For this review, take the finished solid that the model builds, in its own axes (mm). Face numbers are marked on the shaded views. Coordinates: 2 decimals unless noted, no trailing zeros.
from build123d import *

# Parameters (mm, degrees)
SKETCH1_W              = 457.2
SKETCH1_H              = 406.4
BOSS_EXTRUDE1_DEPTH    = 12.7
F_6_CLEARANCE_HOLE1_D  = 3.7973
SKETCH5_R              = 6.4135
CUT_EXTRUDE2_DEPTH     = 307.120058147
CUT_EXTRUDE3_DEPTH     = 3.175
F_10_CLEARANCE_HOLE1_D = 5.1054
CUT_EXTRUDE4_DEPTH     = 307.120058147
FILLET1_R              = 6.35
F_10_CLEARANCE_HOLE2_D = 5.1054
SKETCH18_R             = 6.985
CUT_EXTRUDE6_DEPTH     = 4.7625


with BuildPart() as part:
    # Sketch1 → Boss-Extrude1 (new body)
    with BuildSketch(Plane(origin=(0, 0, 0), x_dir=(1, 0, 0), z_dir=(0, 1, 0))):
        Rectangle(SKETCH1_W, SKETCH1_H)
    extrude(amount=BOSS_EXTRUDE1_DEPTH)

    # #6 Clearance Hole1 (through all)
    with Locations(Plane(origin=(0, 0, 0), x_dir=(-1, 0, 0), z_dir=(0, -1, 0))):
        with Locations((-196.85, 87.87638), (-158.75, 87.87638), (-146.05, 90.45448), (-107.95, 90.45448), (-95.25, 95.83166), (-57.15, 95.83166), (-44.45, 101.50348), (-6.35, 101.50348), (6.35, 107.61726), (44.45, 107.61726), (57.15, 110.71098), (95.25, 110.71098), (107.95, 117.34038), (146.05, 117.34038), (158.75, 124.26442), (196.85, 124.26442), (196.85, -124.26442), (158.75, -124.26442), (146.05, -117.34038), (107.95, -117.34038), (95.25, -110.71098), (57.15, -110.71098), (44.45, -107.61726), (6.35, -107.61726), (-6.35, -101.50348), (-44.45, -101.50348), (-57.15, -95.83166), (-95.25, -95.83166), (-107.95, -90.45448), (-146.05, -90.45448), (-158.75, -87.87638), (-196.85, -87.87638)):
            Hole(F_6_CLEARANCE_HOLE1_D / 2)

    # Sketch5 → Cut-Extrude2 (cut, through all)
    with BuildSketch(Plane.XZ):
        with Locations(Location((0, 0, 0), (0, 0, 270))):
            Circle(SKETCH5_R)
    extrude(amount=-CUT_EXTRUDE2_DEPTH, mode=Mode.SUBTRACT)

    # Sketch6 → Cut-Extrude3 (cut)
    with BuildSketch(Plane.XZ):
        Polygon((-192.913, -121.99139199), (-196.85, -119.71836398), (-200.787, -121.99139199), (-200.787, -126.53744801), (-196.85, -128.81047602), (-192.913, -126.53744801), align=None)
    cut_extrude3 = extrude(amount=-CUT_EXTRUDE3_DEPTH, mode=Mode.SUBTRACT)

    # Sketch-Pattern1: Cut-Extrude3 at 31 more places
    with Locations((393.7, 0, 36.38804), (355.6, 0, 36.38804), (342.9, 0, 33.80994), (304.8, 0, 33.80994), (292.1, 0, 28.43276), (254, 0, 28.43276), (241.3, 0, 22.76094), (203.2, 0, 22.76094), (190.5, 0, 16.64716), (152.4, 0, 16.64716), (139.7, 0, 13.55344), (101.6, 0, 13.55344), (88.9, 0, 6.92404), (50.8, 0, 6.92404), (38.1, 0, 0), (0, 0, 248.52884), (38.1, 0, 248.52884), (50.8, 0, 241.6048), (88.9, 0, 241.6048), (101.6, 0, 234.9754), (139.7, 0, 234.9754), (152.4, 0, 231.88168), (190.5, 0, 231.88168), (203.2, 0, 225.7679), (241.3, 0, 225.7679), (254, 0, 220.09608), (292.1, 0, 220.09608), (304.8, 0, 214.7189), (342.9, 0, 214.7189), (355.6, 0, 212.1408), (393.7, 0, 212.1408)):
        add(cut_extrude3, mode=Mode.SUBTRACT)

    # #10 Clearance Hole1 (through all)
    with Locations(Plane(origin=(0, 12.7, 0), x_dir=(1, 0, 0), z_dir=(0, 1, 0))):
        with Locations((-30.245937227, -17.4625), (0, 34.925), (30.245937227, -17.4625)):
            Hole(F_10_CLEARANCE_HOLE1_D / 2)

    # Sketch10 → Cut-Extrude4 (cut, through all)
    with BuildSketch(Plane(origin=(0, 12.7, 0), x_dir=(1, 0, 0), z_dir=(0, 1, 0))):
        Polygon((67.035234154, -203.2), (228.6, -171.45), (228.6, -203.2), align=None)
        Polygon((228.6, 203.2), (67.035234154, 203.2), (228.6, 171.45), align=None)
    extrude(amount=-CUT_EXTRUDE4_DEPTH, mode=Mode.SUBTRACT)

    # Fillet1
    fillet1_edges = [part.edges().sort_by_distance(p)[0] for p in [
        (67.035234154, 6.35, 203.2),
        (228.6, 6.35, 171.45),
        (228.6, 6.35, -171.45),
        (67.035234154, 6.35, -203.2),
        (-228.6, 6.35, 203.2),
        (-228.6, 6.35, -203.2),
    ]]
    fillet(fillet1_edges, radius=FILLET1_R)

    # #10 Clearance Hole2 (through all)
    with Locations(Plane(origin=(0, 12.7, 0), x_dir=(1, 0, 0), z_dir=(0, 1, 0))):
        with Locations((177.8, -129.661378082), (-177.8, -152.4), (-177.8, 152.4), (177.8, 129.661378082)):
            Hole(F_10_CLEARANCE_HOLE2_D / 2)

    # Sketch18 → Cut-Extrude6 (cut)
    with BuildSketch(Plane.XZ):
        with Locations(Location((-196.85, -124.26442, 0), (0, 0, 270))):
            Circle(SKETCH18_R)
    cut_extrude6 = extrude(amount=-CUT_EXTRUDE6_DEPTH, mode=Mode.SUBTRACT)

    # Sketch-Pattern2: Cut-Extrude6 at 31 more places
    with Locations((393.7, 0, 36.38804), (355.6, 0, 36.38804), (342.9, 0, 33.80994), (304.8, 0, 33.80994), (292.1, 0, 28.43276), (254, 0, 28.43276), (241.3, 0, 22.76094), (203.2, 0, 22.76094), (190.5, 0, 16.64716), (152.4, 0, 16.64716), (139.7, 0, 13.55344), (101.6, 0, 13.55344), (88.9, 0, 6.92404), (50.8, 0, 6.92404), (38.1, 0, 0), (0, 0, 248.52884), (38.1, 0, 248.52884), (50.8, 0, 241.6048), (88.9, 0, 241.6048), (101.6, 0, 234.9754), (139.7, 0, 234.9754), (152.4, 0, 231.88168), (190.5, 0, 231.88168), (203.2, 0, 225.7679), (241.3, 0, 225.7679), (254, 0, 220.09608), (292.1, 0, 220.09608), (304.8, 0, 214.7189), (342.9, 0, 214.7189), (355.6, 0, 212.1408), (393.7, 0, 212.1408)):
        add(cut_extrude6, mode=Mode.SUBTRACT)


solid = part.part
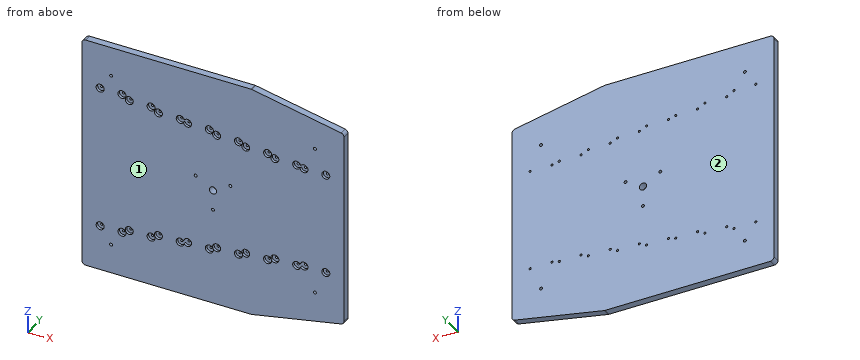
1. Clearance check with flat-ended pins moving along their axes: pin 1 Ø3 at (x, z) = (-13.5, -89.5) entering from -Y; pin 2 Ø7 at (x, z) = (195.5, 87.5) entering from -Y. State where each tip first meets the part, or that it passes through.
Answer below:
pin 1: stops at y = 0
pin 2: stops at y = 4.76
2. The part is to be moulded in two halves that separate along Y. For the marked faces 1 and 2, say which applies: +Y half, -Y half, draft (parallel to the pull), parting line (faces both ways), or undercut.
Answer below:
face 1: -Y half
face 2: +Y half
3. To check wall thickness, follow L1, parallel to Z at x = -57.15, y = 7; L2, parallel to X at y = 8, z = -101; L3, parallel to Z at x = 196.85, y = 10. State the ranges of each line that lie inside material, in increasing order.
Answer below:
L1: z = -203.2 to -112.61, -108.81 to 108.81, 112.61 to 203.2
L2: x = -228.6 to 4.52, 8.18 to 42.62, 46.28 to 228.6
L3: z = -177.69 to -89.78, -85.98 to 85.98, 89.78 to 177.69
4. Take a section at A-A, the plane y = 7.25. Give the number of separate pieces and of enclosed holes in the cut face, plus the area to 3 significant figures.
Answer below:
separate pieces: 1
enclosed holes: 40
area: 180,000 mm2
